Design review of the part built by this model. Coordinates are the model's own, in mm. A direction names the side the tool comes from. Round coordinates to 2 decimals unless told otherwise and drop trailing zeros. Write each loop counter-clockwise with the first axis right and the second up, starting at its lowest first coordinate (ties: lowest second). Pieces come first, ordered by that corner, then holes. Notation, with made-up numbers: (52, 15.25) -> (65, 15.25) arc R12 ccw to (65, 38.25) -> close; hole circle Ø11 at (27, 73). An arc over 180 degrees is marked (long way). One line per question, with ' | ' between items. Start each with the question number.
1) Consider section D-D (z = 82). Give the boundary of the cut face in (x, y) (3 decimals), then the cut area to 3 significant figures.
2) For probe 1 along Z at (x, y) = (64.5, 101.5); probe 2 along X at (y, z) = (40.5, 96); probe 3 along Z at (x, y) = (70, 3.5), list the stretches that pass through material, from the lowest coordinate up.
3) For faces 5 (the flat face through (34.02, -19.64, 112.9)), 6 (the flat face through (69, -14, 62)), 7 (the flat face through (82, 97, 19)), 8 (the flat face through (41.09, 73.584, 245.269)), 9 (the flat face through (73, 97, 38)), list the 3-axis set-ups (+Z, -Z, +X, -X, +Y, -Y) from which the entire face can be reached by the end or side of a thin tool; tool diameter is ignored.
4) Consider section B-B (y = 94.5). Give the boundary of the cut face in (x, z), then the cut area to 3 significant figures.
5) Insertion check: pin 1 Ø15 at (x, z) = (74, 48) entering from +Y; pin 2 Ø11 at (y, z) = (-17.5, 39.5) entering from +X; pin 3 Ø8 at (x, y) = (72, 1.5) entering from +Z. Each pin has a flat end and moves straight along its axis. Give the tip position at first contact, or say it passes through.
6) Mouldability with a two-part tool opening along Z and no side actions: class faces 1 (the flat face through (8.174, 46.543, 245.269)), 2 (the flat face through (53, 44, 151)), 3 (the flat face through (63, 97, 55)), 4 (the flat face through (73, 70.738, 55)) as +Z half, -Z half, draft (parallel to the pull), parting line (faces both ways), or undercut.
7) Consider section A-A (z = 224). Give the boundary of the cut face in (x, y), then the cut area to 3 significant figures.
8) Consider section C-C (x = 31). Give the boundary of the cut face in (y, z), then the cut area to 3 significant figures.
```python
from build123d import *

# Parameters (mm, degrees)
BOSS_EXTRUDE1_DEPTH = 229
BOSS_EXTRUDE3_DEPTH = 33
CUT_EXTRUDE1_DEPTH  = 78
SKETCH4_W           = 33
SKETCH4_H           = 53.425
CUT_EXTRUDE2_DEPTH  = 19
CUT_EXTRUDE3_DEPTH  = 13


with BuildPart() as part:
    # Sketch1 → Boss-Extrude1 (new body)
    with BuildSketch(Plane.XY):
        with BuildLine():
            Line((0, 42.162831426), (0, 0))
            Line((0, 0), (69, -39.837168574))
            Line((69, -39.837168574), (82, -39.837168574))
            Line((82, -39.837168574), (82, 13.587831426))
            ThreePointArc((82, 13.587831426), (53.425, 42.162831426), (82, 70.737831426))
            Line((82, 70.737831426), (82, 124.162831426))
            ThreePointArc((82, 124.162831426), (24.017243943, 100.145587483), (0, 42.162831426))
        make_face()
    extrude(amount=BOSS_EXTRUDE1_DEPTH)

    # Sketch2 → Boss-Extrude3 (add)
    with BuildSketch(Plane.XY.offset(229)):
        with BuildLine():
            Line((50.218978157, 117.75361559), (65.979193229, 105.440386084))
            Line((65.979193229, 105.440386084), (15.494952252, 40.823504288))
            Line((15.494952252, 40.823504288), (0.644773941, 52.425735154))
            ThreePointArc((0.644773941, 52.425735154), (16.616037222, 91.779593848), (50.218978157, 117.75361559))
        make_face()
    extrude(amount=BOSS_EXTRUDE3_DEPTH)

    # Sketch3 → Cut-Extrude1 (cut)
    with BuildSketch(Plane.XY.offset(229)):
        with BuildLine():
            Line((82, 84.108352132), (82, 2.108352132))
            ThreePointArc((82, 2.108352132), (41, 43.108352132), (82, 84.108352132))
        make_face()
    extrude(amount=-CUT_EXTRUDE1_DEPTH, mode=Mode.SUBTRACT)

    # Sketch4 → Cut-Extrude2 (cut)
    with BuildSketch(Plane(origin=(82, 0, 0), x_dir=(0, 0, -1), z_dir=(1, 0, 0))):
        with Locations((-54.5, 97.450331426)):
            Rectangle(SKETCH4_W, SKETCH4_H)
    extrude(amount=-CUT_EXTRUDE2_DEPTH, mode=Mode.SUBTRACT)

    # Sketch5 → Cut-Extrude3 (cut)
    with BuildSketch(Plane(origin=(82, 0, 0), x_dir=(0, 0, -1), z_dir=(1, 0, 0))):
        with BuildLine():
            Line((0, -24.837168574), (-114, -24.837168574))
            ThreePointArc((-114, -24.837168574), (-125, -13.837168574), (-114, -2.837168574))
            Line((-114, -2.837168574), (0, -2.837168574))
            ThreePointArc((0, -2.837168574), (11, -13.837168574), (0, -24.837168574))
        make_face()
    extrude(amount=-CUT_EXTRUDE3_DEPTH, mode=Mode.SUBTRACT)


solid = part.part
```
From the geometry:
1) outline: (0, 0) -> (69, -39.837) -> (82, -39.837) -> (82, -24.837) -> (69, -24.837) -> (69, -2.837) -> (82, -2.837) -> (82, 13.588) arc R28.575 cw to (82, 70.738) -> (82, 124.163) arc R82 ccw to (0, 42.163) -> close | area: 9,060 mm2
2) probe 1: z = 0 to 38, 71 to 229 | probe 2: x = 0 to 53.47 | probe 3: z = 0 to 229
3) face 5: +Z, -Z, -X, -Y | face 6: -Z, +X | face 7: +Z, -Z, +X, +Y, -Y | face 8: +Z, +X, -Y | face 9: +X, +Y
4) outline: (18.77, 229) -> (18.87, 229) -> (18.87, 0) -> (82, 0) -> (82, 38) -> (63, 38) -> (63, 71) -> (82, 71) -> (82, 229) -> (57.43, 229) -> (57.43, 262) -> (18.77, 262) -> close | area: 15,100 mm2
5) pin 1: stops at y = 70.74 | pin 2: stops at x = 69 | pin 3: stops at z = 229
6) face 1: draft | face 2: +Z half | face 3: undercut | face 4: undercut
7) outline: (0, 0) -> (69, -39.84) -> (82, -39.84) -> (82, 2.11) arc R41 cw to (82, 84.11) -> (82, 124.16) arc R82 ccw to (0, 42.16) -> close | area: 7,990 mm2
8) outline: (-17.9, 0) -> (106.37, 0) -> (106.37, 229) -> (106.45, 229) -> (106.45, 262) -> (60.67, 262) -> (60.67, 229) -> (-17.9, 229) -> close | area: 30,000 mm2
